Geometry: final body of the model. Coordinates: model frame, mm. Face numbers are marked on the shaded views. A direction names the side the tool comes from. Coordinates: 2 decimals unless noted, no trailing zeros. Loops run counter-clockwise (first coordinate to the right, second up) from the corner with the lowest first, then second, coordinate; pieces in that order, holes last. Notation, with made-up numbers: M -4,83 L 35,83 A5 cw 35,88 Z; hole C -40,67 d5. An arc over 180 degrees is marked long. Write each question's results on one line, items separated by ' | '. Start each with the question number.
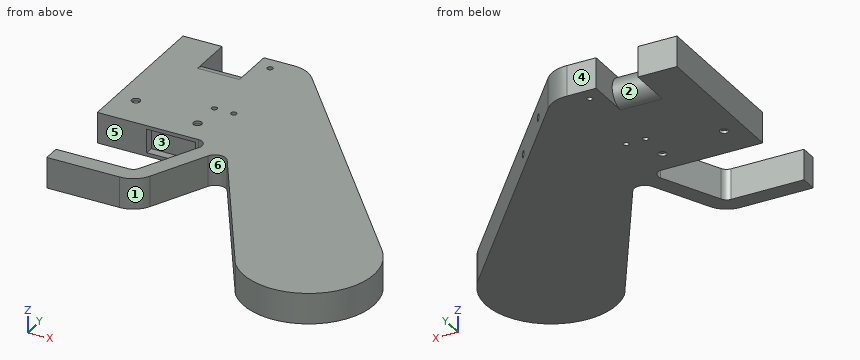
from build123d import *

# Parameters (mm, degrees)
F0_R      = 1
F1_DEPTH  = 5.5
F3_DEPTH  = 25
F4_R      = 1
F5_DEPTH  = 11.001
F6_W      = 17.5
F6_H      = 8.5
F7_DEPTH  = 3
F8_R      = 1.25
F9_DEPTH  = 2
F10_R     = 1.5
F11_DEPTH = 1
F12_R     = 1.5
F13_DEPTH = 1


with BuildPart() as f1:
    # F0 (on Top) → F1 (new body, symmetric)
    with BuildSketch(Plane.XY):
        with BuildLine():
            Line((0, 56), (0, 0))
            Line((0, 0), (36.2259279858, 0))
            ThreePointArc((36.2259279858, 0), (38.7660402441, -1.4038077448), (38.9289329951, -4.3014468563))
            Line((38.9289329951, -4.3014468563), (28.817821884, -25.3014468563))
            ThreePointArc((28.817821884, -25.3014468563), (27.7110091299, -26.5401122582), (26.1148168747, -27))
            Line((26.1148168747, -27), (0, -27))
            Line((0, -27), (0, -33))
            Line((0, -33), (26.1148168747, -33))
            ThreePointArc((26.1148168747, -33), (30.9033936403, -31.6203367747), (34.2238319025, -27.904340569))
            Line((34.2238319025, -27.904340569), (43.9565924234, -7.690145641))
            ThreePointArc((43.9565924234, -7.690145641), (47.3319268627, -5.59281579), (50.7608266635, -7.6013777725))
            Line((50.7608266635, -7.6013777725), (84.9360533184, -64.560088864))
            ThreePointArc((84.9360533184, -64.560088864), (118.0198171676, -67.4369378944), (120.8966661979, -34.3531740452))
            Line((120.8966661979, -34.3531740452), (48.4995788875, 51.8338346577))
            ThreePointArc((48.4995788875, 51.8338346577), (44.4862343011, 54.9569066089), (39.5090393722, 56))
            Line((39.5090393722, 56), (29, 56))
            Line((29, 56), (29, 40))
            Line((29, 40), (14, 40))
            Line((14, 40), (14, 56))
            Line((14, 56), (0, 56))
        make_face()
        with Locations((34, 51)):
            Circle(F0_R, mode=Mode.SUBTRACT)
    extrude(amount=F1_DEPTH, both=True)

    # F2 (on face) → F3 (join)
    with BuildSketch(Plane(origin=(29, 0, 0), x_dir=(0, -1, 0), z_dir=(-1, 0, 0))):
        with BuildLine():
            ThreePointArc((-40, 5.5), (-45.5, 0), (-40, -5.5))
            Line((-40, -5.5), (-40, 5.5))
        make_face()
    extrude(amount=F3_DEPTH)

    # F4 (on face) → F5 (cut, through all)
    with BuildSketch(Plane.XY.offset(5.5)):
        with Locations((31, 20)):
            Circle(F4_R)
        with Locations((38, 20)):
            Circle(F4_R)
    extrude(amount=-F5_DEPTH, mode=Mode.SUBTRACT)

    # F6 (on face) → F7 (cut)
    with BuildSketch(Plane.XZ):
        with Locations((26.4759279858, 0)):
            Rectangle(F6_W, F6_H)
    extrude(amount=-F7_DEPTH, mode=Mode.SUBTRACT)

    # F8 (on face) → F9 (cut)
    with BuildSketch(Plane(origin=(53.9634146341, 45.3292682927, 0), x_dir=(-0.6431920864, 0.7657048648, 0), z_dir=(0.7657048648, 0.6431920864, 0))):
        with Locations((-31.5051259772, 0)):
            Circle(F8_R)
        with Locations((-7.5051259772, 0)):
            Circle(F8_R)
    extrude(amount=-F9_DEPTH, mode=Mode.SUBTRACT)

    # F10 (on face) → F11 (cut)
    with BuildSketch(Plane.XY.offset(5.5)):
        with Locations((7, 12.5)):
            Circle(F10_R)
        with Locations((31, 9)):
            Circle(F10_R)
    extrude(amount=-F11_DEPTH, mode=Mode.SUBTRACT)

    # F12 (on face) → F13 (cut)
    with BuildSketch(Plane(origin=(0, 0, -5.5), x_dir=(1, 0, 0), z_dir=(0, 0, -1))):
        with Locations((7, -12.5)):
            Circle(F12_R)
        with Locations((31, -9)):
            Circle(F12_R)
    extrude(amount=-F13_DEPTH, mode=Mode.SUBTRACT)


solid = f1.part
Item 1: Section D-D, the plane x = 78. Return loops of the section in (y, z), plus the area to 3 significant figures.
Item 2: Section C-C, the plane y = 4.5. Return loops of the section in (x, z), plus the area to 3 significant figures.
Item 3: Contact query for flat-ended pins moving along their axis: P1, Ø3, axis at y = 21.5, z = -3, coming from the -X side; P2, Ø3.5, axis at y = 2, z = -1, coming from the +X side; P3, Ø3.5, axis at x = 4.5, z = 1.5, coming from the +Y side; P4, Ø1.6, axis at x = 31, y = 20, coming from the +Z side. Output: stop coordinate, or through.
Item 4: Set-up query: the marked faces 1, 2 and 3. Return all of +Z, -Z, +X, -X, +Y, -Y with unobstructed straight access to the full face (end or side cutting, diameter ignored); none if empty.
Item 5: Section B-B, the plane y = -17. Return loops of the section in (x, z).
Item 6: Section A-A, the plane x = 7. Return loops of the section in (y, z), plus the area to 3 significant figures.
Item 7: Ray query, L1, parallel to Y at x = 38, z = -2.75; L2, parallel to X at y = -24.5, z = -2.25; L3, parallel to X at y = 9, z = -5. Return the intervals inside material, ascending. Write a range as [from, to].
Item 8: Pull-direction query (Y, two-part tool) for the marked faces 4, 5 and 6; classes: released by +Y, released by -Y, zero draft, split by the parting line, or undercut.
Solutions:
1) outline: M -53,-5.5 L 16.71,-5.5 L 16.71,5.5 L -53,5.5 Z | area: 767 mm²
2) outline: M 0,-5.5 L 88.26,-5.5 L 88.26,5.5 L 0,5.5 Z | area: 971 mm²
3) P1: stops at x = 0 | P2: stops at x = 91.83 | P3: stops at y = 56 | P4: passes through
4) face 1: +Z, -Z, -Y | face 2: +Y | face 3: none
5) outline: M 32.81,-5.5 L 39.47,-5.5 L 39.47,5.5 L 32.81,5.5 Z; M 56.4,-5.5 L 106.32,-5.5 L 106.32,5.5 L 56.4,5.5 Z
6) outline: M -33,-5.5 L -27,-5.5 L -27,5.5 L -33,5.5 Z; M 0,-5.5 L 11,-5.5 L 11,-4.5 L 14,-4.5 L 14,-5.5 L 56,-5.5 L 56,5.5 L 14,5.5 L 14,4.5 L 11,4.5 L 11,5.5 L 0,5.5 Z | area: 676 mm²
7) L1: y = [-20.06, -6.23], [-0.58, 19], [21, 56] | L2: x = [29.2, 35.86], [60.9, 112.62] | L3: x = [0, 29.5], [32.5, 84.48]
8) face 4: released by +Y | face 5: undercut | face 6: released by -Y
